Build history of the part. All positions in model axes, mm. A direction names the side the tool comes from. Give positions to 0.01 mm unless a question says otherwise; leave off trailing zeros. Write each loop counter-clockwise with the first axis right and the second up, starting at its lowest first coordinate (ties: lowest second). Pieces come first, ordered by that corner, then holes. Notation, with made-up numbers: (-38, 68) - (-19, 68) arc R28 ccw to (-19, 105) - close; hole circle Ø8 at (47.5, -12). An arc over 180 degrees is marked (long way). Use one line per item in the form item = value. Start each with the question number.
Autodesk Inventor part; units mm, degrees
ref_plane "YZ Plane" through (0, 0, 0) normal (1, 0, 0) x (0, 1, 0)
ref_plane "XZ Plane" through (0, 0, 0) normal (0, 1, 0) x (-1, 0, 0)
ref_plane "XY Plane" through (0, 0, 0) normal (0, 0, 1) x (1, 0, 0)
sketch "Sketch1" plane through (0, 0, 0) normal (0, 0, 1) x (1, 0, 0)
  line L0 (0, 0) -> (50.8, 0)
  line L1 (50.8, 0) -> (50.8, 25.4)
  line L2 (50.8, 25.4) -> (25.4, 25.4)
  line L3 (25.4, 25.4) -> (25.4, 63.5)
  line L4 (25.4, 63.5) -> (0, 63.5)
  line L5 (0, 63.5) -> (0, 0)
  dimension "d0" = 50.8
  dimension "d2" = 25.4
  dimension "d3" = 25.4
  dimension "d4" = 38.1
extrude "Extrusion1" add sketch "Sketch1" along normal blind 3.175
sketch "Sketch2" plane through (0, 0, 0) normal (0, 0, -1) x (-1, 0, 0)
  circle A0 centre (-38.1, 12.7) radius 3.3782
  circle A1 centre (-12.7, 48.0173) radius 3.302
  circle A2 centre (4.1663, 34.7761) radius 4.4593
sketch "Sketch3" plane through (0, 0, 0) normal (0, 0, -1) x (-1, 0, 0)
  line L0 (0, 0) -> (-50.8, 0)
  line L1 (0, 63.5) -> (0, 0)
  line L2 (-25.4, 63.5) -> (0, 63.5)
  line L3 (-25.4, 25.4) -> (-25.4, 63.5)
  line L4 (-50.8, 25.4) -> (-25.4, 25.4)
  line L5 (-50.8, 0) -> (-50.8, 25.4)
  circle A0 centre (-38.1, 12.7) radius 3.3782
  line L6 (-22.225, 38.6193) -> (-22.225, 32.0153)
  circle A1 centre (-38.1, 12.7) radius 3.3782
extrude "Extrusion2" cut sketch "Sketch2" against normal blind 25.4 contours A0 | A1
properties part number "ninja"
(1) Cut at C-C, the plane z = 2.4. Give the cut face in (x, y).
(2) Two-plate mould, pull along X, no slides. Class faces 1 (the flat face through (50.8, 13, 2)), 2 (the flat face through (25, 0, 2)), 3 (the cylindrical face through (15.134, 50.249, 1.565)): +X half, -X half, draft (parallel to the pull), parting line (faces both ways), or undercut.
(3) Cut at B-B, the plane y = 12.7. Give the cut face in (x, z) (3 decimals).
(4) Cut at D-D, the plane x = 31.5. Give the cut face in (y, z) (3 decimals).
(5) Cut at A-A, the plane x = 38.1. Give the cut face in (y, z) (3 decimals).
(6) Which spindle directions (+Z, -Z, +X, -X, +Y, -Y) get a long thin tool onto all of the face, cutting with end or side? Do faces 4 (the flat face through (38, 25.4, 2)), 5 (the flat face through (19, 25, 3.175)). Say none if no direction does.
(7) Pin check, flat tips, straight feed: pin 1 Ø1.6 at (y, z) = (38.5, 2.5) entering from +X; pin 2 Ø1.6 at (x, z) = (42, 1.5) entering from +Y; pin 3 Ø6 at (x, y) = (12.7, 48.02) entering from +Z. Stop position of each tip, or through.
(8) Wall check: line 1 (Y direction, x = 38.1, z = 2.45); line 2 (Y direction, x = 13, z = 2.9); line 3 (Y direction, x = 29, z = 0.55). Give the ranges that are in metal, low to high. Write a range as from..to.
Solution:
q1.outline = (0, 0) - (50.8, 0) - (50.8, 25.4) - (25.4, 25.4) - (25.4, 63.5) - (0, 63.5) - close; hole circle Ø6.6 at (12.7, 48.02); hole circle Ø6.76 at (38.1, 12.7)
q2.face_1 = +X half
q2.face_2 = draft
q2.face_3 = undercut
q3.outline = (0, 0) - (34.722, 0) - (34.722, 3.175) - (0, 3.175) - close; (41.478, 0) - (50.8, 0) - (50.8, 3.175) - (41.478, 3.175) - close
q4.outline = (0, 0) - (25.4, 0) - (25.4, 3.175) - (0, 3.175) - close
q5.outline = (0, 0) - (9.322, 0) - (9.322, 3.175) - (0, 3.175) - close; (16.078, 0) - (25.4, 0) - (25.4, 3.175) - (16.078, 3.175) - close
q6.face_4 = +Z, -Z, +X, +Y
q6.face_5 = +Z, +X, -X, +Y, -Y
q7.pin_1 = 25.4
q7.pin_2 = 25.4
q7.pin_3 = through
q8.line_1 = 0..9.32, 16.08..25.4
q8.line_2 = 0..44.73, 51.31..63.5
q8.line_3 = 0..25.4
